Check sheet for the modelled part. Datum: model origin and axes. Units: mm. Give positions to 0.01 mm unless a question says otherwise; leave off trailing zeros. Write each loop counter-clockwise with the first axis right and the second up, starting at its lowest first coordinate (ties: lowest second). Pieces come first, ordered by that corner, then holes.
from build123d import *

# Parameters (mm, degrees)
PAD003_DEPTH = 2.5
FILLET002_R  = 1
FILLET003_R  = 0.3


with BuildPart() as part:
    # Sketch033 (on Face94 of Binder) → Pad003 (new body)
    with BuildSketch(Plane(origin=(1.8936722157, -3.2799364905, 0), x_dir=(0.8660254038, 0.5, 0), z_dir=(0.5, -0.8660254038, 0))):
        with BuildLine():
            Line((-10.53, 58.8773011628), (-14.13, 58.8773011628))
            Line((-14.13, 58.8773011628), (-14.13, 21))
            Line((-14.13, 21), (-10.53, 21))
            Line((-10.53, 36), (-10.53, 21))
            ThreePointArc((-10.13, 36), (-10.33, 36.2), (-10.53, 36))
            Line((-10.13, 21), (-10.13, 36))
            Line((-10.13, 21), (-10.13, 18.5))
            Line((-10.13, 18.5), (-11.13, 18.5))
            Line((-11.13, 18.5), (-9.93, 15))
            Line((-9.93, 15), (-7.33, 15))
            Line((-7.33, 15), (-7.33, 36))
            ThreePointArc((-6.33, 36), (-6.83, 36.5), (-7.33, 36))
            Line((-6.33, 36), (-6.33, 15))
            Line((-6.33, 15), (6.07, 15))
            Line((6.07, 15), (6.07, 36))
            ThreePointArc((7.07, 36), (6.57, 36.5), (6.07, 36))
            Line((7.07, 36), (7.07, 15))
            Line((7.07, 15), (9.67, 15))
            Line((9.67, 15), (10.87, 18.5))
            Line((10.87, 18.5), (9.87, 18.5))
            Line((9.87, 21), (9.87, 18.5))
            Line((9.87, 21), (9.87, 36))
            ThreePointArc((10.27, 36), (10.07, 36.2), (9.87, 36))
            Line((10.27, 36), (10.27, 21))
            Line((13.87, 21), (10.27, 21))
            Line((13.87, 58.8773011628), (13.87, 21))
            Line((10.27, 58.8773011628), (13.87, 58.8773011628))
            Line((10.27, 43.8773011628), (10.27, 58.8773011628))
            ThreePointArc((9.87, 43.8773011628), (10.07, 43.6773011628), (10.27, 43.8773011628))
            Line((9.87, 58.8773011628), (9.87, 43.8773011628))
            Line((9.87, 61.3773011628), (9.87, 58.8773011628))
            Line((10.87, 61.3773011628), (9.87, 61.3773011628))
            Line((9.67, 64.8773011628), (10.87, 61.3773011628))
            Line((7.07, 64.8773011628), (9.67, 64.8773011628))
            Line((7.07, 43.8773011628), (7.07, 64.8773011628))
            ThreePointArc((6.07, 43.8773011628), (6.57, 43.3773011628), (7.07, 43.8773011628))
            Line((6.07, 64.8773011628), (6.07, 43.8773011628))
            Line((-6.33, 64.8773011628), (6.07, 64.8773011628))
            Line((-6.33, 43.8773011628), (-6.33, 64.8773011628))
            ThreePointArc((-7.33, 43.8773011628), (-6.83, 43.3773011628), (-6.33, 43.8773011628))
            Line((-7.33, 64.8773011628), (-7.33, 43.8773011628))
            Line((-9.93, 64.8773011628), (-7.33, 64.8773011628))
            Line((-11.13, 61.3773011628), (-9.93, 64.8773011628))
            Line((-10.13, 61.3773011628), (-11.13, 61.3773011628))
            Line((-10.13, 58.8773011628), (-10.13, 61.3773011628))
            Line((-10.13, 58.8773011628), (-10.13, 43.8773011628))
            ThreePointArc((-10.53, 43.8773011628), (-10.33, 43.6773011628), (-10.13, 43.8773011628))
            Line((-10.53, 43.8773011628), (-10.53, 58.8773011628))
        make_face()
    extrude(amount=PAD003_DEPTH)

    # Fillet002
    fillet002_edges = [part.edges().sort_by_distance(p)[0] for p in [
        (10.893138, 0.472532, 15),
        (-6.08096, -9.327468, 15),
        (-6.08096, -9.327468, 64.877301),
        (10.893138, 0.472532, 64.877301),
    ]]
    fillet(fillet002_edges, radius=FILLET002_R)

    # Fillet003
    fillet003_edges = [part.edges().sort_by_distance(p)[0] for p in [
        (11.932368, 1.072532, 18.5),
        (-7.120191, -9.927468, 18.5),
        (-7.120191, -9.927468, 61.377301),
        (11.932368, 1.072532, 61.377301),
    ]]
    fillet(fillet003_edges, radius=FILLET003_R)


solid = part.part
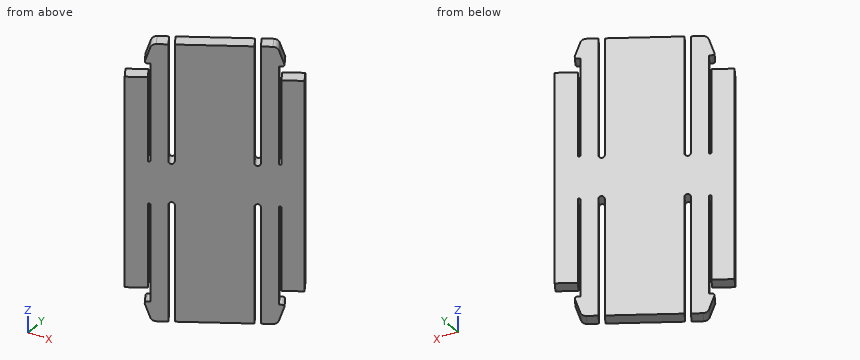
1) Sectioned sample at C-C on x = 4. Record the boundary of the cut face in (y, z).
2) Scan lines: L1, parallel to X at y = -1.25, z = 56.5; L2, parallel to X at y = 0, z = 49; L3, parallel to Y at x = 5.5, z = 24.5. Record each from-to range of solid material in increasing order.
3) Sectioned sample at B-B on z = 41.5. Record the boundary of the cut face in (x, y).
4) Gauge pin test, flat ends, axial feed: pin 1 (1 mm diameter, centred on y = -2.5, z = 51, fed in from +X); pin 2 (2 mm diameter, centred on y = -1, z = 36, fed in from -X); pin 3 (4.5 mm diameter, centred on x = 12.5, y = 1, fed in from -Z). Record the tip position at first contact, or that the pin passes through.
5) Sectioned sample at A-A on z = 30. Record the boundary of the cut face in (x, y), then the cut area to 3 significant figures.
Answers below:
1. outline: (-4.95, 15) - (-2.06, 15) - (-2.06, 64.88) - (-4.95, 64.88) - close
2. L1: x = 5.41 to 7.73, 8.89 to 10.41
2. L2: x = 8.16 to 11.4, 11.86 to 12.57
2. L3: y = -4.08 to -1.2
3. outline: (-10.34, -10.34) - (-9.09, -12.51) - (15.16, 1.49) - (13.91, 3.66) - close
4. pin 1: stops at x = 8.4
4. pin 2: stops at x = 4.11
4. pin 3: stops at z = 15.01
5. outline: (-10.34, -10.34) - (-9.09, -12.51) - (-5.98, -10.71) - (-7.23, -8.54) - close; (-6.88, -8.34) - (-5.63, -10.51) - (-3.2, -9.11) - (-4.45, -6.94) - close; (-3.59, -6.44) - (-2.34, -8.61) - (8.4, -2.41) - (7.15, -0.24) - close; (8.02, 0.26) - (9.27, -1.91) - (11.69, -0.51) - (10.44, 1.66) - close; (10.79, 1.86) - (12.04, -0.31) - (15.16, 1.49) - (13.91, 3.66) - close
5. area: 63.0 mm2
